```python
from build123d import *

# Parameters (mm, degrees)
F1_DEPTH  = 12.7
F2_W      = 12.7
F2_H      = 12.7
F3_DEPTH  = 114.3
F4_W      = 12.7
F4_H      = 12.7
F5_DEPTH  = 177.8
F6_W      = 12.7
F6_H      = 12.7
F7_DEPTH  = 177.8
F8_W      = 12.7
F8_H      = 12.7
F9_DEPTH  = 685.8
F10_W     = 12.7
F10_H     = 12.7
F11_DEPTH = 685.8
F12_W     = 10.16
F12_H     = 10.16
F13_DEPTH = 254.001
F14_W     = 10.16
F14_H     = 10.16
F15_DEPTH = 190.501
F16_W     = 10.16
F16_H     = 10.16
F17_DEPTH = 254.001


with BuildPart() as f1:
    # F0 (on Top) → F1 (new body)
    with BuildSketch(Plane.XY):
        Polygon((0, 254), (0, 0), (12.7, 0), (12.7, 241.3), (698.5, 241.3), (698.5, 0), (711.2, 0), (711.2, 254), align=None)
    extrude(amount=F1_DEPTH)

    # F2 (on face) → F3 (join)
    with BuildSketch(Plane.XY.offset(12.7)):
        with Locations((6.35, 247.65)):
            Rectangle(F2_W, F2_H)
        with Locations((704.85, 247.65)):
            Rectangle(F2_W, F2_H)
    extrude(amount=F3_DEPTH)

    # F4 (on face) → F5 (join)
    with BuildSketch(Plane.XZ.offset(-241.3)):
        with Locations((6.35, 120.65)):
            Rectangle(F4_W, F4_H)
    extrude(amount=F5_DEPTH)

    # F6 (on face) → F7 (join)
    with BuildSketch(Plane.XZ.offset(-241.3)):
        with Locations((704.85, 120.65)):
            Rectangle(F6_W, F6_H)
    extrude(amount=F7_DEPTH)

    # F8 (on face) → F9 (join, through all)
    with BuildSketch(Plane.YZ.offset(12.7)):
        with Locations((247.65, 120.65)):
            Rectangle(F8_W, F8_H)
    extrude(amount=F9_DEPTH)

    # F10 (on face) → F11 (join, through all)
    with BuildSketch(Plane.YZ.offset(12.7)):
        with Locations((69.85, 120.65)):
            Rectangle(F10_W, F10_H)
    extrude(amount=F11_DEPTH)

    # F12 (on face) → F13 (cut, through all)
    with BuildSketch(Plane.XZ):
        with Locations((704.85, 6.35)):
            Rectangle(F12_W, F12_H)
    extrude(amount=-F13_DEPTH, mode=Mode.SUBTRACT)

    # F14 (on face) → F15 (cut, through all)
    with BuildSketch(Plane.XZ.offset(-63.5)):
        with Locations((704.85, 120.65)):
            Rectangle(F14_W, F14_H)
        with Locations((6.35, 120.65)):
            Rectangle(F14_W, F14_H)
    extrude(amount=-F15_DEPTH, mode=Mode.SUBTRACT)

    # F16 (on face) → F17 (cut, through all)
    with BuildSketch(Plane.XZ):
        with Locations((6.35, 6.35)):
            Rectangle(F16_W, F16_H)
    extrude(amount=-F17_DEPTH, mode=Mode.SUBTRACT)


solid = f1.part
```
Source: CAD feature listing. Evaluate the final solid. Frame: model axes, mm. A direction names the side the tool comes from. Round coordinates to 2 decimals unless told otherwise and drop trailing zeros. Write each loop counter-clockwise with the first axis right and the second up, starting at its lowest first coordinate (ties: lowest second). Pieces come first, ordered by that corner, then holes. Notation, with made-up numbers: M 71.25,63.5 L 126.25,63.5 A19 ccw 126.25,95.5 Z; hole C -38.5,41 d1. An arc over 180 degrees is marked long. Use CSV: the item, a comma, the result in double quotes. Start each with the question number.
Q1. Cut plane D-D on z = 95. Output: boundary loops of the cut face in (x, y).
Q2. Cut plane C-C on y = 94. Count the separate pieces of the cut face and the enclosed holes in it, plus the area to 3 significant figures.
Q3. Pull-direction query (X, two-part tool) for faces 1 (the face through (6, 122, 12.7)), 2 (the face through (351, 248, 12.7)), 3 (the face through (12.7, 160, 121)); classes: +X half, -X half, draft (parallel to the pull), parting line (faces both ways), or undercut.
Q4. Cut plane B-B on x = 469.5. Output: boundary loops of the cut face in (y, z), plus the area to 3 significant figures.
Q5. Cut plane A-A on y = 42.5. Output: boundary loops of the cut face in (x, z), plus the area to 3 significant figures.
Q6. Access query for faces 4 (the face through (12.7, 248, 63)), 5 (the face through (6, 241.3, 63)), 6 (the face through (351, 241.3, 6)), 7 (the face through (301, 254, 11)), 8 (the face through (351, 76.2, 121)). Directions: +Z, -Z, +X, -X, +Y, -Y. A direction counts if a zero-diameter tool reaches every point of the face in a straight line with its end or side. Return the directions, or none.
Q7. First-contact query: P1, Ø6, axis at x = 76.5, z = 18, coming from the +Y side; P2, Ø10, axis at x = 706, z = 45, coming from the -Y side; P3, Ø10, axis at x = 362.5, z = 122.5, coming from the -Y side. Flat tips, straight axial feed; report the tip coordinate or a pass-through.
Q8. Line query: line 1 (X direction, y = 137, z = 116.5); line 2 (Y direction, x = 242, z = 121.5); line 3 (Z direction, x = 274, y = 75). Output: solid intervals per line, ascending. Write a range as from..to.
Results found:
1,outline,"M 0,241.3 L 12.7,241.3 L 12.7,254 L 0,254 Z; M 698.5,241.3 L 711.2,241.3 L 711.2,254 L 698.5,254 Z"
2,separate pieces,"4"
2,enclosed holes,"4"
2,area,"232 mm^2"
3,face 1,"draft"
3,face 2,"undercut"
3,face 3,"undercut"
4,outline,"M 63.5,114.3 L 76.2,114.3 L 76.2,127 L 63.5,127 Z; M 241.3,0 L 254,0 L 254,12.7 L 241.3,12.7 Z; M 241.3,114.3 L 254,114.3 L 254,127 L 241.3,127 Z"
4,area,"484 mm^2"
5,outline,"M 0,0 L 12.7,0 L 12.7,12.7 L 0,12.7 Z; M 698.5,0 L 711.2,0 L 711.2,12.7 L 698.5,12.7 Z; hole M 1.27,1.27 L 11.43,1.27 L 11.43,11.43 L 1.27,11.43 Z; hole M 699.77,1.27 L 709.93,1.27 L 709.93,11.43 L 699.77,11.43 Z"
5,area,"116 mm^2"
6,face 4,"+Y, -Y"
6,face 5,"+X, -X, -Y"
6,face 6,"+Z, -Z, -Y"
6,face 7,"+Z, -Z, +X, -X, +Y"
6,face 8,"+Z, -Z"
7,P1,"through"
7,P2,"y = 241.3"
7,P3,"y = 63.5"
8,line 1,"0..1.27, 11.43..12.7, 698.5..699.77, 709.93..711.2"
8,line 2,"63.5..76.2, 241.3..254"
8,line 3,"114.3..127"
